```python
from build123d import *

# Parameters (mm, degrees)
SKETCH1_R           = 2.5
BOSS_EXTRUDE1_DEPTH = 4


with BuildPart() as part:
    # Sketch1 → Boss-Extrude1 (new body)
    with BuildSketch(Plane.XY):
        with BuildLine():
            Line((2, -4), (2, 1.120548597))
            add(Edge.make_bspline(
                [(2, 1.120548597), (7.835899457, 4.971392719), (6, 12)],
                knots=[0.134548696, 0.134548696, 0.134548696, 1, 1, 1], degree=2))
            Line((6, 12), (3, 12))
            Line((3, 12), (3, 10))
            Line((3, 10), (-3, 10))
            Line((-3, 10), (-3, 12))
            Line((-3, 12), (-6, 12))
            add(Edge.make_bspline(
                [(-2, 1.120548597), (-7.835899457, 4.971392719), (-6, 12)],
                knots=[0.134548696, 0.134548696, 0.134548696, 1, 1, 1], degree=2))
            Line((-2, 1.120548597), (-2, -4))
            Line((-2, -4), (2, -4))
        make_face()
        with Locations((0, 7)):
            Circle(SKETCH1_R, mode=Mode.SUBTRACT)
    extrude(amount=BOSS_EXTRUDE1_DEPTH)


solid = part.part
```
The model under review builds one solid part; all positions refer to its coordinate system, in mm. A direction names the side the tool comes from. Round coordinates to 2 decimals unless told otherwise and drop trailing zeros. Write each loop counter-clockwise with the first axis right and the second up, starting at its lowest first coordinate (ties: lowest second). Pieces come first, ordered by that corner, then holes. Notation, with made-up numbers: M 2,54 L 8,54 A24 cw 8,74 Z; hole C 73.25,84.25 d6. An arc over 180 degrees is marked long. Use CSV: the item, a comma, the result in double quotes. Start each with the question number.
(1) Clearance check with flat-ended pins moving along their axes: P1, Ø4.5, axis at x = 0, y = 7, coming from the +Z side; P2, Ø2, axis at y = -0.5, z = 3, coming from the +X side; P3, Ø1.6, axis at y = 11, z = 2, coming from the +X side; P4, Ø0.6, axis at y = 11.5, z = 2, coming from the -X side. State where each tip first meets the part, or that it passes through.
(2) For line 1 along Y through (x, z) = (0, 2.25); line 2 along X through (y, z) = (0, 3.8); line 3 along X through (y, z) = (6, 2.95), list the stretches that pass through material, from the lowest coordinate up.
(3) We need section A-A, the plane x = 0. State the section outline as (y, z) points, then the cut area to 3 significant figures.
(4) The part is to be moulded in two halves that separate along X. For faces 4 (the face through (0, 10, 2)), 5 (the face through (2, -1, 2)), 6 (the face through (-4, 12, 2)), say which applies: +X half, -X half, draft (parallel to the pull), parting line (faces both ways), or undercut.
(5) Tool access review of faces 1 (the face through (-3, 11, 2)), 2 (the face through (5, 12, 2)), 3 (the face through (-2, -1, 2)): name each direction out of +Z, -Z, +X, -X, +Y, -Y from which nothing blocks a thin tool from reaching the whole face with its end or side.
Findings:
1,P1,"through"
1,P2,"x = 2"
1,P3,"x = 6.35"
1,P4,"x = -6.19"
2,line 1,"-4 to 4.5, 9.5 to 10"
2,line 2,"-2 to 2"
2,line 3,"-6 to -2.29, 2.29 to 6"
3,outline,"M -4,0 L 4.5,0 L 4.5,4 L -4,4 Z; M 9.5,0 L 10,0 L 10,4 L 9.5,4 Z"
3,area,"36.0 mm^2"
4,face 4,"undercut"
4,face 5,"+X half"
4,face 6,"draft"
5,face 1,"+Z, -Z, +Y"
5,face 2,"+Z, -Z, +X, -X, +Y"
5,face 3,"+Z, -Z, -X, -Y"
